Could you check a few things on this model? Use its own coordinates, in mm. Give positions to 0.01 mm unless a question says otherwise; leave off trailing zeros. Loops run counter-clockwise (first coordinate to the right, second up) from the corner with the lowest first, then second, coordinate; pieces in that order, holes last. Notation, with made-up numbers: (78.25, -34.75) - (134.25, -34.75) arc R24 cw to (134.25, -9.75) - close; hole circle Ø6 at (16, 85). An arc over 180 degrees is marked (long way). Write each question's results on one line, items separated by ' | '. Start each with the question number.
1) I want a section at D-D, the plane z = 3.5. Write out the boundary of the cut face in (x, y), and give its area (3 significant figures).
2) I want a section at C-C, the plane y = 0.55. Write out the boundary of the cut face in (x, z), and give its area (3 significant figures).
3) I'm going to push flat-ended pins straight in: pin 1 (10.5 mm diameter, centred on x = 42.07, z = 26.19, fed in from +Y); pin 2 (1 mm diameter, centred on x = 20.5, y = 0.5, fed in from -Z); pin 3 (5 mm diameter, centred on x = -42.07, z = 26.19, fed in from -Y); pin 4 (4 mm diameter, centred on x = 15.5, z = -21, fed in from +Y). Where does each tip first touch, or does it pass through?
4) If I drill on probe 1 along X at (y, z) = (1.55, 14.5); probe 2 along X at (y, z) = (1.8, 22.5); probe 3 along X at (y, z) = (0.3, -25.5), over which ranges is the centre line in solid material (lowest first)? Write a range as [from, to].
5) I want a section at A-A, the plane x = 28. Write out the boundary of the cut face in (y, z), and give its area (3 significant figures).
6) I want a section at B-B, the plane z = -12.5. Write out the boundary of the cut face in (x, y).
Solid Edge part; units mm, degrees
sketch "Sketch1" plane through (0, 0, 0) normal (0, -1, 0) x (1, 0, 0)
  line L0 (48, 32) -> (-48, 32)
  line L1 (-48, 32) -> (-48, -32)
  line L2 (-48, -32) -> (48, -32)
  line L3 (48, -32) -> (48, 32)
extrude "Protrusion1" add sketch "Sketch1" against normal blind 2
hole "Hole_1" at (-42.0687, 0, 26.1937) direction (0, 1, 0) diameter 3.175 end up to next counterbore diameter 6.604 counterbore depth 1
hole "Hole1" at (42.0688, 0, 26.1937) direction (0, 1, 0) diameter 3.175 end up to next counterbore diameter 6.604 counterbore depth 1
hole "Hole2" at (42.0688, 0, -26.1938) direction (0, 1, 0) diameter 3.175 end up to next counterbore diameter 6.604 counterbore depth 1
hole "Hole3" at (-42.0687, 0, -26.1938) direction (0, 1, 0) diameter 3.175 end up to next counterbore diameter 6.604 counterbore depth 1
sketch "Sketch2" plane through (0, 0, 0) normal (0, -1, 0) x (1, 0, 0)
  line L0 (59.2211, 38.1609) -> (-59.2211, 38.1609)
  line L1 (-59.2211, 38.1609) -> (-59.2211, -38.4291)
  line L2 (-59.2211, -38.4291) -> (59.2211, -38.4291)
  line L3 (59.2211, -38.4291) -> (59.2211, 38.1609)
  line L4 (-38.9763, 31.1079) -> (-4.9726, 9.7098)
  arc A0 (-4.9726, 9.7098) -> (4.9726, 9.7098) centre (0, -0.1341) cw
  line L5 (38.9763, 31.1079) -> (4.9726, 9.7098)
  line L6 (10.9467, -0.0838) -> (45.1439, 21.2687)
  line L7 (45.1766, -21.1419) -> (10.9467, -0.0838)
  line L8 (38.9274, -31.2248) -> (4.932, -9.9983)
  line L9 (-38.9274, -31.2248) -> (-4.932, -9.9983)
  line L10 (-45.1766, -21.1419) -> (-10.9467, -0.0838)
  line L11 (-10.9467, -0.0838) -> (-45.1439, 21.2687)
  arc A1 (38.9763, 31.1078) -> (45.1439, 21.2687) centre (42.0688, 26.1937) cw
  arc A2 (45.1766, -21.1419) -> (38.9275, -31.2247) centre (42.0688, -26.1937) cw
  arc A3 (4.932, -9.9983) -> (-4.932, -9.9983) centre (0, -0.1341) cw
  arc A4 (-38.9274, -31.2248) -> (-45.1765, -21.142) centre (-42.0687, -26.1938) cw
  arc A5 (-45.1439, 21.2687) -> (-38.9763, 31.108) centre (-42.0687, 26.1937) cw
extrude "Cutout1" cut sketch "Sketch2" against normal blind 174.286
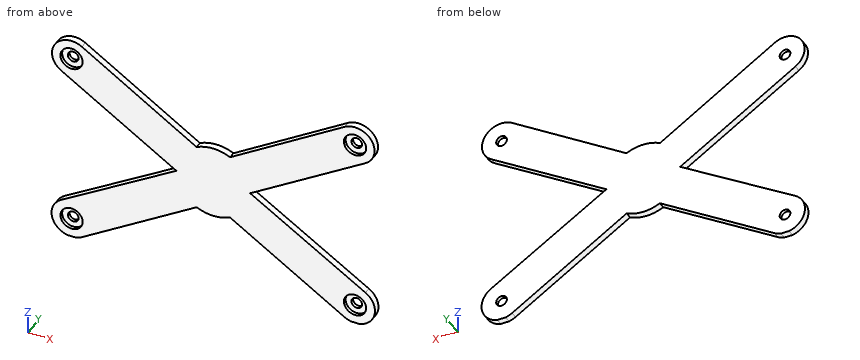
Answers:
1) outline: (-16.69, 0) - (16.69, 0) - (16.69, 2) - (-16.69, 2) - close | area: 66.7 mm2
2) outline: (-45.18, -21.14) arc R5.93 ccw to (-43.28, -32) - (-40.86, -32) arc R5.93 ccw to (-38.93, -31.22) - (-4.93, -10) arc R11.03 ccw to (4.93, -10) - (38.93, -31.22) arc R5.93 ccw to (40.86, -32) - (43.28, -32) arc R5.93 ccw to (45.18, -21.14) - (10.95, -0.08) - (45.14, 21.27) arc R5.81 ccw to (38.98, 31.11) - (4.97, 9.71) arc R11.03 ccw to (-4.97, 9.71) - (-38.98, 31.11) arc R5.81 ccw to (-45.14, 21.27) - (-10.95, -0.08) - close; hole circle Ø6.6 at (-42.07, -26.19); hole circle Ø6.6 at (-42.07, 26.19); hole circle Ø6.6 at (42.07, -26.19); hole circle Ø6.6 at (42.07, 26.19) | area: 2,280 mm2
3) pin 1: stops at y = 2 | pin 2: stops at z = -20.03 | pin 3: stops at y = 1 | pin 4: passes through
4) probe 1: x = [-34.3, -12.58], [12.58, 34.3] | probe 2: x = [-46.55, -25.3], [25.3, 46.55] | probe 3: x = [-47.96, -45.3], [-38.84, -29.76], [29.76, 38.84], [45.3, 47.96]
5) outline: (0, -24.4) - (2, -24.4) - (2, -10.57) - (0, -10.57) - close; (0, 10.56) - (2, 10.56) - (2, 24.2) - (0, 24.2) - close | area: 54.9 mm2
6) outline: (-31.13, 0) - (-8.94, 0) - (-8.94, 2) - (-31.13, 2) - close; (8.94, 0) - (31.13, 0) - (31.13, 2) - (8.94, 2) - close
